from build123d import *

# Parameters (mm, degrees)
BASE_FLANGE1_DEPTH   = 304.8
EDGE_FLANGE3_DEPTH   = 53.34
SKETCH14_W           = 20.32
SKETCH14_H           = 69.210930463
CUT_EXTRUDE1_DEPTH   = 9.4615
EDGE_FLANGE4_DEPTH   = 12.7
MIRROR2_COPY_1_DEPTH = 12.7
SKETCH22_W           = 17.803399203
SKETCH22_H           = 9.246782325
SKETCH22_W_2         = 16.822955406
TAB1_DEPTH           = 1.5875


# Sheet-metal steps are written as plain solids
with BuildPart() as part:
    # Sketch1 → Base-Flange1 (new body)
    with BuildSketch(Plane(origin=(0, 0, 0), x_dir=(1, 0, 0), z_dir=(0, 1, 0))):
        with BuildLine():
            Line((19.05, 0), (2.54, 0))
            ThreePointArc((2.54, 0), (0.743948776, 0.743948776), (0, 2.54))
            Line((0, 2.54), (0, 53.34))
            ThreePointArc((0, 53.34), (0.743948776, 55.136051224), (2.54, 55.88))
            Line((2.54, 55.88), (55.88, 55.88))
            ThreePointArc((55.88, 55.88), (57.676051224, 55.136051224), (58.42, 53.34))
            Line((58.42, 53.34), (58.42, 2.54))
            ThreePointArc((58.42, 2.54), (57.676051224, 0.743948776), (55.88, 0))
            Line((55.88, 0), (39.37, 0))
            Line((39.37, 0), (39.37, -1.5875))
            Line((39.37, -1.5875), (55.88, -1.5875))
            ThreePointArc((55.88, -1.5875), (58.798583239, -0.378583239), (60.0075, 2.54))
            Line((60.0075, 2.54), (60.0075, 53.34))
            ThreePointArc((60.0075, 53.34), (58.798583239, 56.258583239), (55.88, 57.4675))
            Line((55.88, 57.4675), (2.54, 57.4675))
            ThreePointArc((2.54, 57.4675), (-0.378583239, 56.258583239), (-1.5875, 53.34))
            Line((-1.5875, 53.34), (-1.5875, 2.54))
            ThreePointArc((-1.5875, 2.54), (-0.378583239, -0.378583239), (2.54, -1.5875))
            Line((2.54, -1.5875), (19.05, -1.5875))
            Line((19.05, -1.5875), (19.05, 0))
        make_face()
    extrude(amount=BASE_FLANGE1_DEPTH)

    # Edge-Flange3 section (across the edge) → Edge-Flange3 (add)
    with BuildSketch(Plane(origin=(2.54, -7.874, -55.88), x_dir=(0, 1, 0), z_dir=(1, 0, 0))):
        with BuildLine():
            Line((-1.5875, 2.54), (-1.5875, 56.8325))
            Line((-1.5875, 56.8325), (0, 56.8325))
            Line((0, 56.8325), (0, 2.54))
            ThreePointArc((0, 2.54), (0.743948776, 0.743948776), (2.54, 0))
            Line((2.54, 0), (7.874, 0))
            Line((7.874, 0), (7.874, -1.5875))
            Line((7.874, -1.5875), (2.54, -1.5875))
            ThreePointArc((2.54, -1.5875), (-0.378583239, -0.378583239), (-1.5875, 2.54))
        make_face()
    extrude(amount=EDGE_FLANGE3_DEPTH)

    # Sketch14 → Cut-Extrude1 (cut)
    with BuildSketch(Plane.XZ.offset(9.4615)):
        with Locations((29.21, -26.70801644)):
            Rectangle(SKETCH14_W, SKETCH14_H)
    extrude(amount=-CUT_EXTRUDE1_DEPTH, mode=Mode.SUBTRACT)

    # Edge-Flange4 section (across the edge) → Edge-Flange4 (add)
    with BuildSketch(Plane(origin=(-1.5875, 307.34, -21.59), x_dir=(0, -1, 0), z_dir=(0, 0, -1))):
        with BuildLine():
            Line((-1.5875, 2.54), (-1.5875, 13.97))
            Line((-1.5875, 13.97), (0, 13.97))
            Line((0, 13.97), (0, 2.54))
            ThreePointArc((0, 2.54), (0.743948776, 0.743948776), (2.54, 0))
            Line((2.54, 0), (2.54, -1.5875))
            ThreePointArc((2.54, -1.5875), (-0.378583239, -0.378583239), (-1.5875, 2.54))
        make_face()
    edge_flange4 = extrude(amount=EDGE_FLANGE4_DEPTH)

    # Mirror1: Edge-Flange4 across plane
    add(edge_flange4.mirror(Plane(origin=(29.21, 0, 0), x_dir=(0, 0, 1), z_dir=(1, 0, 0))))

    # Mirror2: Edge-Flange4 across plane
    add(edge_flange4.mirror(Plane.ZX.offset(152.4)))

    # Mirror2 copy 1 sketch → Mirror2 copy 1 (add)
    with BuildSketch(Plane(origin=(60.0075, -2.54, -21.59), x_dir=(0, 1, 0), z_dir=(0, 0, -1))):
        with BuildLine():
            Line((-1.5875, 2.54), (-1.5875, 13.97))
            Line((-1.5875, 13.97), (0, 13.97))
            Line((0, 13.97), (0, 2.54))
            ThreePointArc((0, 2.54), (0.743948776, 0.743948776), (2.54, 0))
            Line((2.54, 0), (2.54, -1.5875))
            ThreePointArc((2.54, -1.5875), (-0.378583239, -0.378583239), (-1.5875, 2.54))
        make_face()
    extrude(amount=MIRROR2_COPY_1_DEPTH)

    # Sketch22 → Tab1 (add)
    with BuildSketch(Plane(origin=(60.0075, 0, 0), x_dir=(0, 0, -1), z_dir=(1, 0, 0))):
        with Locations((11.441699601, -4.623391162)):
            Rectangle(SKETCH22_W, SKETCH22_H)
        with Locations((44.004958561, -4.623391162)):
            Rectangle(SKETCH22_W_2, SKETCH22_H)
    tab1 = extrude(amount=-TAB1_DEPTH)

    # Mirror3: Tab1 across plane
    add(tab1.mirror(Plane(origin=(29.21, 0, 0), x_dir=(0, 0, 1), z_dir=(1, 0, 0))))


solid = part.part
Model file for the job. Use its own axes, mm. A direction names the side the tool comes from. Give positions to 0.01 mm unless a question says otherwise; leave off trailing zeros. Loops run counter-clockwise (first coordinate to the right, second up) from the corner with the lowest first, then second, coordinate; pieces in that order, holes last. Notation, with made-up numbers: (78, 23.25) -> (95, 23.25) arc R23 ccw to (95, 38.25) -> close; hole circle Ø1 at (50, -0.5). An arc over 180 degrees is marked (long way). Use a Markdown table: item, result. Add a question column.
(1) Tool access for faces 4 (the flat face through (39.37, -9, -33)), 5 (the flat face through (59, 304.8, -5)), 6 (the flat face through (11, 150, 0)), 7 (the flat face through (29.1, 304.8, -56.2)), 8 (the flat face through (68, 307.34, -28)): list every direction of +Z, -Z, +X, -X, +Y, -Y with a clear straight run to the whole face (end or side of a thin tool).
(2) Mould opens along Z. For faces 1 (the flat face through (29, 148, -55.88)), 2 (the flat face through (55.88, -8.2, -32.4)), 3 (the flat face through (11, 150, 1.588)) say: +Z half, -Z half, draft (parallel to the pull), parting line (faces both ways), or undercut.
(3) Slice it at B-B on z = -28.5. Give the number of separate pieces and of enclosed holes in the cut face, and give its area (3 significant figures).
(4) Wall check: line 1 along X through (y, z) = (197.5, -24.5); line 2 along Z through (x, y) = (12, 191.5); line 3 along Y through (x, z) = (64.5, -33.5). Give the ranges that are in metal, low to high.
(5) Slice it at A-A on x = 10. List the corners of the cut face in (y, z) (1 decimal).
(6) Drop flat-ended pins along their axis: pin 1 Ø6 at (y, z) = (250, -28) entering from -X; pin 2 Ø1.5 at (x, z) = (16, -8) entering from +Y; pin 3 Ø0.5 at (x, y) = (-1, -4) entering from -Z. Give the stop position or say it passes through.
(7) Slice it at C-C on z = -14. List the corners of the cut face in (x, y), and give its area (3 significant figures).
Filled sheet:
| question | item | result |
|---|---|---|
| 1 | face 4 | +Z, -Z, -Y |
| 1 | face 5 | +Z, +X, -X, +Y |
| 1 | face 6 | +Y |
| 1 | face 7 | -Z, +X, -X, +Y |
| 1 | face 8 | +Z, -Z, +X |
| 2 | face 1 | undercut |
| 2 | face 2 | draft |
| 2 | face 3 | +Z half |
| 3 | separate pieces | 4 |
| 3 | enclosed holes | 0 |
| 3 | area | 1,130 mm2 |
| 4 | line 1 | -1.59 to 0, 58.42 to 60.01 |
| 4 | line 2 | -57.47 to -55.88, 0 to 1.59 |
| 4 | line 3 | -4.13 to -2.54, 307.34 to 308.93 |
| 5 | outline | (-9.5, -53.3) arc R4.1 ccw to (-5.3, -57.5) -> (304.8, -57.5) -> (304.8, -55.9) -> (-5.3, -55.9) arc R2.5 cw to (-7.9, -53.3) -> (-7.9, 1) -> (-9.5, 1) -> close; (0, 0) -> (304.8, 0) -> (304.8, 1.6) -> (0, 1.6) -> close |
| 6 | pin 1 | x = -1.59 |
| 6 | pin 2 | y = -7.87 |
| 6 | pin 3 | z = -52.42 |
| 7 | outline | (-1.59, -9.25) -> (0, -9.25) -> (0, 304.8) -> (-1.59, 304.8) -> close; (2.54, -9.46) -> (19.05, -9.46) -> (19.05, -7.87) -> (2.54, -7.87) -> close; (39.37, -9.46) -> (55.88, -9.46) -> (55.88, -7.87) -> (39.37, -7.87) -> close; (58.42, -9.25) -> (60.01, -9.25) -> (60.01, 304.8) -> (58.42, 304.8) -> close |
| 7 | area | 1,050 mm2 |
